Autodesk Inventor part; units mm, degrees
ref_plane "Work Plane1" through (60, 0, 0) normal (0, 0, 1) x (1, 0, 0)
ref_plane "YZ Plane" through (0, 0, 0) normal (1, 0, 0) x (0, 1, 0)
ref_plane "XZ Plane" through (0, 0, 0) normal (0, 1, 0) x (-1, 0, 0)
sketch "Sketch1" plane through (0, 0, 0) normal (0, 0, 1) x (1, 0, 0)
  line L0 (0, 2.3) -> (0, 1.5)
  line L1 (0, 1.5) -> (16, 1.5)
  line L2 (16, 1.5) -> (16, 0)
  line L3 (16, 0) -> (-0.4001, 0)
  line L4 (-3.6801, 0) -> (19.28, 0)
  line L5 (-0.4001, 0) -> (-0.4001, 2.3)
  line L6 (-0.4001, 2.3) -> (0, 2.3)
  line L7 (0, -0.46) -> (0, 2.76)
  dimension "d0" = 16
  dimension "d1" = 3
  dimension "d8" = 0.4001
  dimension "d9" = 4.6
revolve "Body" add sketch "Sketch1" angle 360 about axis through (16, 0, 0) along (-1, 0, 0)
sketch "Sketch2" plane through (-0.4001, 0, 0) normal (-1, 0, 0) x (0, 0, 1)
  line L0 (0, 3.1754) -> (2.75, 1.5877)
  line L1 (2.75, 1.5877) -> (2.75, -1.5877)
  line L2 (2.75, -1.5877) -> (0, -3.1754)
  line L3 (0, -3.1754) -> (-2.75, -1.5877)
  line L4 (-2.75, -1.5877) -> (-2.75, 1.5877)
  line L5 (-2.75, 1.5877) -> (0, 3.1754)
  point P0 (0, 0)
  point P1 (0, 0)
  dimension "d10" = 5.5
extrude "Head" add sketch "Sketch2" along normal blind 1.6
sketch "Sketch3" plane through (0, 0, 0) normal (0, 0, 1) x (1, 0, 0)
  line L0 (-2.0001, 0.4) -> (-1.3001, 0.4)
  line L1 (-1.3001, 0.4) -> (-1.3001, -0.4)
  line L2 (-1.3001, -0.4) -> (-2.0001, -0.4)
  line L3 (-2.0001, -0.4) -> (-2.0001, 0.4)
  line L4 (-1.3001, 0) -> (-2.0001, 0) construction
  line L5 (-2.1401, 0) -> (-1.1601, 0)
  line L6 (-2.0001, 1.5877) -> (-2.0001, -1.5877)
  dimension "d11" = 0.8
  dimension "d13" = 0.7
extrude "Slot" cut sketch "Sketch3" along normal through all both and the other way through all
sketch "Sketch4" plane through (0, 0, 0) normal (0, 0, 1) x (1, 0, 0)
  line L0 (-2.0001, 2.75) -> (-2.0001, 3.1754)
  line L1 (-2.0001, 3.1754) -> (-1.7545, 3.1754)
  line L2 (-1.7545, 3.1754) -> (-2.0001, 2.75)
  line L3 (-1.7545, 3.1754) -> (-2.0001, 3.1754)
  line L4 (-2.0001, 3.1754) -> (-2.0001, 2.75)
  line L5 (-2.0001, 3.1754) -> (-2.0001, 1.5877)
  line L6 (-2.3201, 0) -> (-0.0801, 0)
  line L7 (-0.4001, 3.1754) -> (-2.0001, 3.1754)
  dimension "d4" = 30
  dimension "d17" = 5.5
revolve "Chamfer1" cut sketch "Sketch4" angle 360 about axis through (-10, 0, 0) along (1, 0, 0)
thread "Thread"
chamfer "Chamfer2" distance 0.3067 distance2 0.3068 1 edges at (16, -1.5, 0) measured on face at (16, -0.3888, -0.2119)
ref_plane "Work Plane1" through (60, 0, 0) normal (0, 0, 1) x (1, 0, 0)
equation "\"d0\" = NLG"
equation "\"d1\" = GD"
equation "\"d9\" = SD2"
equation "\"d10\" = SW"
equation "\"d2\" = KOH - SD"
equation "\"d11\" = SBR"
equation "\"d13\" = STI"
equation "\"d4\" = ANG1"
equation "\"d17\" = SW0"
equation "\"d15\" = GEL"
equation "\"d5\" = -0.5 * SPD + 0.5 * GD"
equation "\"NLG\" = 16"
equation "\"GD\" = NND"
equation "\"KOH\" = 2"
equation "\"GEL\" = 15.5"
equation "\"SW\" = 5.5"
equation "\"SW0\" = SW"
equation "\"SPD\" = NND - 1.2269 * PTC"
equation "\"SD2\" = SDH"
equation "\"SD\" = WFT"
equation "\"ANG1\" = 30deg"
equation "\"GUL\" = 0.61345 * PTC"
equation "\"STI\" = 0.7"
equation "\"SBR\" = 0.8"
equation "\"RR\" = 0.1"
equation "\"GAL\" = 0.61345 * PTC"
equation "\"BDM\" = NND"
equation "\"WFT\" = 0.4"
equation "\"FAWI\" = 45deg"
equation "\"PTC\" = 0.5"
equation "\"THREADDIA\" = 3"
equation "\"E0\" = 1.155 * SW"
equation "\"TOA\" = 30deg"
equation "\"NND\" = 3"
equation "\"GD1\" = THREADDIA - 1.2269 * PTC"
equation "\"SDH\" = 4.6"
properties part number "Bolt GB 29.1 M3 x 16" material "Acero, suave"
CAD build for the part. Positions are in the model's coordinates, mm. A direction names the side the tool comes from. Give positions to 0.01 mm unless a question says otherwise; leave off trailing zeros. Loops run counter-clockwise (first coordinate to the right, second up) from the corner with the lowest first, then second, coordinate; pieces in that order, holes last. Notation, with made-up numbers: M 25,79.5 L 71,79.5 A28 cw 71,112.5 Z; hole C 27,56 d8. An arc over 180 degrees is marked long. One line per question, with ' | ' between items. Start each with the question number.
1. Two-plate mould, pull along X, no slides. Class faces 3 (the face through (0, 0, 2)), 4 (the face through (-1, 0, -2.75)), 5 (the face through (-2, 1, 0)): pulls with the +X half, pulls with the -X half, needs draft (parallel to the pull), parting line crosses it, or undercut.
2. Saw through at B-B on x = 11. Give the cut face in (y, z).
3. Probe L1, parallel to X at y = 1.5, z = 1.7; L2, parallel to X at y = -2.25, z = -1.35; L3, parallel to Y at x = 8.75, z = -0.1. List the from-to ranges inside material, lowest first. Write a range as from..to.
4. Flat gauge pins, fed straight in: pin 1 (1 mm diameter, centred on y = -0.5, z = -1.5, fed in from +X); pin 2 (2 mm diameter, centred on x = 13, y = -0.5, fed in from -Z); pin 3 (1.5 mm diameter, centred on x = 5.5, y = 0.5, fed in from +Z); pin 4 (0.6 mm diameter, centred on x = -2, z = 1, fed in from +Y). Where does each tip first touch, or does it go through?
5. 3-axis set-ups, long thin cutter, end or side, ignore diameter. For faces 1 (the face through (7.96, -1.5, 0.07)), 2 (the face through (-1.189, 2.37, -1.394)): which of +Z, -Z, +X, -X, +Y, -Y reach the whole face in a straight line?
6. Saw through at A-A on y = 0. Give the cut face in (x, z).
Result sheet:
1) face 3: pulls with the +X half | face 4: needs draft | face 5: pulls with the -X half
2) outline: C 0,0 d3
3) L1: x = -2..0 | L2: x = -2..-0.4 | L3: y = -1.5..1.5
4) pin 1: stops at x = 16 | pin 2: stops at z = -1.5 | pin 3: stops at z = 1.5 | pin 4: stops at y = 2.77
5) face 1: +X | face 2: -Z, +X, -X, +Y
6) outline: M -1.3,-2.75 L -0.4,-2.75 L -0.4,-2.3 L 0,-2.3 L 0,-1.5 L 15.69,-1.5 L 16,-1.19 L 16,1.19 L 15.69,1.5 L 0,1.5 L 0,2.3 L -0.4,2.3 L -0.4,2.75 L -1.3,2.75 Z
